Geometry: final body of the model. Coordinates: model frame, mm. Coordinates: 2 decimals unless noted, no trailing zeros. Order: outer loops, then holes, each group sorted by start corner. A loop starts at its lowest first (then second) coordinate and runs counter-clockwise, first axis right, second up. Notation, with made-up numbers: M 75,44 L 95,44 A20 ccw 95,72 Z; hole C -34,41.25 d11. An arc over 180 degrees is marked long. One line per question, with ' | ' between items.
from build123d import *

# Parameters (mm, degrees)
F0_W          = 340
F0_H          = 70
F1_DEPTH      = 10
F2_R          = 20
F3_R          = 15
F4_DEPTH      = 353
F4_DEPTH_BACK = 25


# Not quite as in the source:
# - an extrude ends at something that could not be found from the text; its depth is read off the source's solid


with BuildPart() as f1:
    # F0 (on Front) → F1 (new body)
    with BuildSketch(Plane.XZ):
        Rectangle(F0_W, F0_H)
    extrude(amount=F1_DEPTH)

    # F2
    f2_edges = [f1.edges().sort_by_distance(p)[0] for p in [
        (-170, -5, 35),
        (-170, -5, -35),
    ]]
    fillet(f2_edges, radius=F2_R)

    # F3 (on Front) → F4 (cut, two sides)
    with BuildSketch(Plane.XZ) as f4_sk:
        with Locations((-135, 0)):
            Circle(F3_R)
        with Locations((-25, 0)):
            Circle(F3_R)
    extrude(amount=-F4_DEPTH, mode=Mode.SUBTRACT)
    extrude(f4_sk.sketch, amount=F4_DEPTH_BACK, mode=Mode.SUBTRACT)


solid = f1.part
1. Section B-B, the plane z = 0. Output: boundary loops of the cut face in (x, y).
Response values:
outline: M -170,-10 L -150,-10 L -150,0 L -170,0 Z; M -120,-10 L -40,-10 L -40,0 L -120,0 Z; M -10,-10 L 170,-10 L 170,0 L -10,0 Z
2. Section C-C, the plane y = -2.25. Output: boundary loops of the cut face in (x, z).
Response values:
outline: M -170,-15 A20 ccw -150,-35 L 170,-35 L 170,35 L -150,35 A20 ccw -170,15 Z; hole C -135,0 d30; hole C -25,0 d30
3. Draft query along X for faces 1 (the face through (-164.297, -5.07, -28.986)), 2 (the face through (-39.985, -4.93, 0.66)), 3 (the face through (-2, -10, 0)). Return one class per face: pulls with the +X half, pulls with the -X half, needs draft (parallel to the pull), parting line crosses it, or undercut.
Response values:
face 1: pulls with the -X half | face 2: undercut | face 3: needs draft
4. Section D-D, the plane x = -25.5. Output: boundary loops of the cut face in (y, z), and give its area (3 significant figures).
Response values:
outline: M -10,-35 L 0,-35 L 0,-14.99 L -10,-14.99 Z; M -10,14.99 L 0,14.99 L 0,35 L -10,35 Z | area: 400 mm^2
5. Section A-A, the plane x = -135. Output: boundary loops of the cut face in (y, z), and give its area (3 significant figures).
Response values:
outline: M -10,-35 L 0,-35 L 0,-15 L -10,-15 Z; M -10,15 L 0,15 L 0,35 L -10,35 Z | area: 400 mm^2
6. Material intervals for line 1 (X direction, y = -5, z = 0); line 2 (X direction, y = -7, z = -10); line 3 (Z direction, x = -135, y = -5.75), sorted ascending. Write a range as [from, to].
Response values:
line 1: x = [-170, -150], [-120, -40], [-10, 170] | line 2: x = [-170, -146.18], [-123.82, -36.18], [-13.82, 170] | line 3: z = [-35, -15], [15, 35]
7. Pin query (flat end, axial travel): P1, Ø18, axis at x = -135, z = 0, coming from the +Y side. Return the tip coordinate at first contact, or that it passes through.
Response values:
P1: passes through
